Check sheet for the modelled part. Datum: model origin and axes. Units: mm. Face numbers are marked on the shaded views. Round coordinates to 2 decimals unless told otherwise and drop trailing zeros. Answer in a Markdown table with one row per item.
Autodesk Inventor part; units mm, degrees
ref_plane "Work Plane1" through (0, 0, 101.6) normal (0, 0, 1) x (1, 0, 0)
ref_plane "Work Plane2" through (0, 0, 98.425) normal (0, 0, 1) x (1, 0, 0)
ref_plane "YZ Plane" through (0, 0, 0) normal (1, 0, 0) x (0, 1, 0)
sketch "Sketch1" plane through (0, 0, 0) normal (0, 0, 1) x (1, 0, 0)
  line L0 (-251.1425, 0) -> (251.1425, 0) construction
  line L1 (0, -146.685) -> (0, 146.685) construction
  line L2 (-179.3875, 104.775) -> (179.3875, 104.775)
  line L3 (179.3875, 104.775) -> (179.3875, -104.775)
  line L4 (179.3875, -104.775) -> (-179.3875, -104.775)
  line L5 (-179.3875, -104.775) -> (-179.3875, 104.775)
  point P0 (0, 0)
  point P1 (0, 104.775)
  point P2 (-179.3875, 0)
  dimension "d0" = 358.775
  dimension "d1" = 209.55
ref_plane "Work Plane1" through (0, 0, 101.6) normal (0, 0, 1) x (1, 0, 0)
sketch "Sketch2" plane through (0, 0, 101.6) normal (0, 0, 1) x (1, 0, 0)
  line L0 (0, -146.685) -> (0, 146.685) construction
  line L1 (-253.365, 0) -> (253.365, 0) construction
  line L2 (-128.5875, 53.975) -> (128.5875, 53.975)
  line L3 (128.5875, 53.975) -> (128.5875, -53.975)
  line L4 (128.5875, -53.975) -> (-128.5875, -53.975)
  line L5 (-128.5875, -53.975) -> (-128.5875, 53.975)
  line L6 (-179.3875, 104.775) -> (179.3875, 104.775) construction
  line L7 (-179.3875, -104.775) -> (-179.3875, 104.775) construction
  point P0 (0, 0)
  point P1 (0, 53.975)
  point P2 (-128.5875, 0)
  dimension "d3" = 50.8
  dimension "d4" = 50.8
loft "Loft1" add profiles "Sketch1", "Sketch2"
sketch "Sketch3" plane through (179.3875, 104.775, 0) normal (0, 0, -1) x (-1, 0, 0)
  line L0 (179.3875, -251.46) -> (179.3875, 41.91) construction
  line L1 (430.53, -104.775) -> (-71.755, -104.775) construction
  line L2 (3.175, -3.175) -> (28.575, -3.175) construction
  line L3 (355.6, -3.175) -> (355.6, -28.575) construction
  line L4 (355.6, -206.375) -> (330.2, -206.375) construction
  line L5 (3.175, -206.375) -> (3.175, -180.975) construction
  line L6 (28.575, -3.175) -> (28.575, -28.575)
  line L7 (28.575, -28.575) -> (3.175, -28.575)
  line L8 (3.175, -180.975) -> (28.575, -180.975)
  line L9 (28.575, -180.975) -> (28.575, -206.375)
  line L10 (330.2, -3.175) -> (330.2, -28.575)
  line L11 (330.2, -28.575) -> (355.6, -28.575)
  line L12 (330.2, -206.375) -> (330.2, -180.975)
  line L13 (330.2, -180.975) -> (355.6, -180.975)
  line L14 (3.175, -28.575) -> (3.175, -3.175) construction
  line L15 (28.575, -3.175) -> (330.2, -3.175)
  line L16 (330.2, -3.175) -> (355.6, -3.175) construction
  line L17 (355.6, -28.575) -> (355.6, -180.975)
  line L18 (355.6, -180.975) -> (355.6, -206.375) construction
  line L19 (330.2, -206.375) -> (28.575, -206.375)
  line L20 (28.575, -206.375) -> (3.175, -206.375) construction
  line L21 (3.175, -180.975) -> (3.175, -28.575)
  line L22 (0, 0) -> (0, -209.55) construction
  line L23 (358.775, 0) -> (0, 0) construction
  point P0 (179.3875, -104.775)
  point P1 (179.3875, -3.175)
  point P2 (3.175, -104.775)
  dimension "d9" = 3.175
  dimension "d10" = 3.175
  dimension "d11" = 25.4
ref_plane "Work Plane2" through (0, 0, 98.425) normal (0, 0, 1) x (1, 0, 0)
sketch "Sketch5" plane through (0, 0, 98.425) normal (0, 0, 1) x (1, 0, 0)
  line L0 (150.8125, 101.6) -> (150.8125, 76.2)
  line L1 (150.8125, 76.2) -> (176.2125, 76.2)
  line L2 (176.2125, -76.2) -> (176.2125, 76.2)
  line L3 (176.2125, -76.2) -> (150.8125, -76.2)
  line L4 (150.8125, -76.2) -> (150.8125, -101.6)
  line L5 (-150.8125, -101.6) -> (150.8125, -101.6)
  line L6 (-150.8125, -101.6) -> (-150.8125, -76.2)
  line L7 (-150.8125, -76.2) -> (-176.2125, -76.2)
  line L8 (-176.2125, 76.2) -> (-176.2125, -76.2)
  line L9 (-150.8125, 76.2) -> (-176.2125, 76.2)
  line L10 (-150.8125, 101.6) -> (-150.8125, 76.2)
  line L11 (150.8125, 101.6) -> (-150.8125, 101.6)
  line L12 (-100.0125, 50.8) -> (-100.0125, 25.4)
  line L13 (-100.0125, 25.4) -> (-125.4125, 25.4)
  line L14 (-125.4125, 25.4) -> (-125.4125, -25.4)
  line L15 (-125.4125, -25.4) -> (-100.0125, -25.4)
  line L16 (-100.0125, -25.4) -> (-100.0125, -50.8)
  line L17 (-100.0125, -50.8) -> (100.0125, -50.8)
  line L18 (100.0125, -50.8) -> (100.0125, -25.4)
  line L19 (100.0125, -25.4) -> (125.4125, -25.4)
  line L20 (125.4125, -25.4) -> (125.4125, 25.4)
  line L21 (125.4125, 25.4) -> (100.0125, 25.4)
  line L22 (100.0125, 25.4) -> (100.0125, 50.8)
  line L23 (100.0125, 50.8) -> (-100.0125, 50.8)
  line L24 (-128.5875, 53.975) -> (128.5875, 53.975)
  point P0 (0, 0)
  dimension "d15" = 3.175
loft "Loft2" cut profiles "Sketch3", "Sketch5" contours all / L23 L22 L21 L20 L19 L18 L17 L16 L15 L14 L13 L12
sketch "Sketch6" plane through (179.3875, 104.775, 0) normal (0, 0, -1) x (-1, 0, 0)
  line L0 (430.53, -104.775) -> (-71.755, -104.775) construction
  line L1 (179.3875, -251.46) -> (179.3875, 41.91) construction
  line L2 (15.875, -15.875) -> (342.9, -15.875) construction
  line L3 (342.9, -15.875) -> (342.9, -193.675) construction
  line L4 (342.9, -193.675) -> (15.875, -193.675) construction
  line L5 (15.875, -193.675) -> (15.875, -15.875) construction
  line L6 (3.175, -28.575) -> (28.575, -28.575) construction
  line L7 (28.575, -28.575) -> (28.575, -3.175) construction
  circle A0 centre (15.875, -15.875) radius 3.175
  circle A1 centre (342.9, -15.875) radius 3.175
  circle A2 centre (342.9, -193.675) radius 3.175
  circle A3 centre (15.875, -193.675) radius 3.175
  point P0 (179.3875, -104.775)
  point P1 (179.3875, -15.875)
  point P2 (15.875, -104.775)
  dimension "d20" = 12.7
  dimension "d21" = 12.7
  dimension "d22" = 6.35
extrude "Extrusion1" cut sketch "Sketch6" against normal through all
equation "\"d21\" = d20"
properties part number "Front Cover"
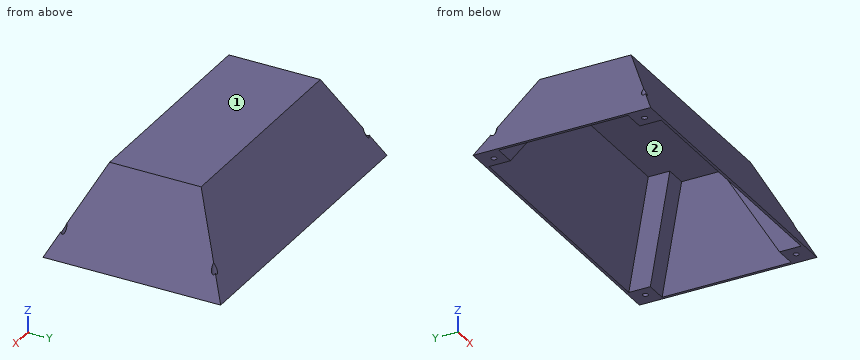
(1) Depth check by flat-ended pin: pin 1 Ø10 at (y, z) = (14, 65) entering from -X; pin 2 Ø10 at (x, y) = (163.51, -88.9) entering from +Z; pin 3 Ø12 at (x, z) = (4, 68.5) entering from +Y (3 decimals); pin 4 Ø5.5 at (x, y) = (163.51, 88.9) entering from -Z. Enter the tip coordinate at first touch or a pass-through.
Solutions:
| item | result |
|---|---|
| pin 1 | x = -149.39 |
| pin 2 | z = 38.82 |
| pin 3 | y = 73.525 |
| pin 4 | through |
(2) Draft check along Y on the marked faces 1 and 2. Enter one of: pulls with the +Y half, pulls with the -Y half, needs draft (parallel to the pull), parting line crosses it, or undercut.
Solutions:
| item | result |
|---|---|
| face 1 | needs draft |
| face 2 | undercut |
(3) Scan lines: probe 1 along X at (y, z) = (-88, 21); probe 2 along X at (y, z) = (88, 12); probe 3 along Z at (x, y) = (-43, 2) (3 decimals). Record each from-to range of solid material in increasing order. Write a range as from..to.
Solutions:
| item | result |
|---|---|
| probe 1 | -168.89..-166.56, -160.47..-139.97, 139.97..160.47, 166.56..168.89 |
| probe 2 | -173.39..-166.56, -160.47..-144.62, 144.62..160.47, 166.56..173.39 |
| probe 3 | 98.425..101.6 |
